```python
from build123d import *

# Parameters (mm, degrees)
SKETCH_1_R          = 23
SKETCH_1_R_2        = 20
EXTRUDE_1_DEPTH     = 20
SKETCH_2_W          = 10
SKETCH_2_H          = 19.630909826
CUT_EXTRUDE_1_DEPTH = 20
SKETCH_3_W          = 5
SKETCH_3_H          = 10
EXTRUDE_2_DEPTH     = 20
FILLET_1_R          = 2
SKETCH_4_R          = 2.15
CUT_EXTRUDE_2_DEPTH = 20
SKETCH_5_W          = 8
SKETCH_5_H          = 11
EXTRUDE_3_DEPTH     = 20
SKETCH_6_R          = 1.5
CUT_EXTRUDE_3_DEPTH = 23


with BuildPart() as part:
    # 草图1 → 凸台-拉伸1 (new body)
    with BuildSketch(Plane.XY):
        Circle(SKETCH_1_R)
        Circle(SKETCH_1_R_2, mode=Mode.SUBTRACT)
    extrude(amount=EXTRUDE_1_DEPTH)

    # 草图2 → 切除-拉伸1 (cut)
    with BuildSketch(Plane.XY.offset(20)):
        with Locations((0, -20)):
            Rectangle(SKETCH_2_W, SKETCH_2_H)
    extrude(amount=-CUT_EXTRUDE_1_DEPTH, mode=Mode.SUBTRACT)

    # 草图3 → 凸台-拉伸2 (add)
    with BuildSketch(Plane.XY.offset(20)):
        with Locations((-7.5, -24.364916731)):
            Rectangle(SKETCH_3_W, SKETCH_3_H)
        with Locations((7.5, -24.364916731)):
            Rectangle(SKETCH_3_W, SKETCH_3_H)
    extrude(amount=-EXTRUDE_2_DEPTH)

    # 圆角1
    fillet_1_edges = [part.edges().sort_by_distance(p)[0] for p in [
        (5, -19.364916731, 10),
        (-5, -19.364916731, 10),
    ]]
    fillet(fillet_1_edges, radius=FILLET_1_R)

    # 草图4 → 切除-拉伸2 (cut)
    with BuildSketch(Plane(origin=(10, 0, 0), x_dir=(0, 0, -1), z_dir=(1, 0, 0))):
        with Locations(Location((-15, -25.038615954, 0), (0, 0, 90))):
            Circle(SKETCH_4_R)
        with Locations(Location((-5, -25.038615954, 0), (0, 0, 90))):
            Circle(SKETCH_4_R)
    extrude(amount=-CUT_EXTRUDE_2_DEPTH, mode=Mode.SUBTRACT)

    # 草图5 → 凸台-拉伸3 (add)
    with BuildSketch(Plane(origin=(0, 0, 0), x_dir=(-1, 0, 0), z_dir=(0, 0, -1))):
        with Locations((0, 27.5)):
            Rectangle(SKETCH_5_W, SKETCH_5_H)
    extrude(amount=-EXTRUDE_3_DEPTH)

    # 草图6 → 切除-拉伸3 (cut)
    with BuildSketch(Plane(origin=(4, 0, 0), x_dir=(0, 0, -1), z_dir=(1, 0, 0))):
        with Locations(Location((-5, 28, 0), (0, 0, 90))):
            Circle(SKETCH_6_R)
        with Locations(Location((-15, 28, 0), (0, 0, 90))):
            Circle(SKETCH_6_R)
    extrude(amount=-CUT_EXTRUDE_3_DEPTH, mode=Mode.SUBTRACT)


solid = part.part
```
Source: CAD feature listing. Evaluate the final solid. Frame: model axes, mm. A direction names the side the tool comes from. Coordinates: 2 decimals unless noted, no trailing zeros. Order: outer loops, then holes, each group sorted by start corner. A loop starts at its lowest first (then second) coordinate and runs counter-clockwise, first axis right, second up. Notation, with made-up numbers: (78, -14) - (102, -14) arc R33 ccw to (102, 16) - close; hole circle Ø2 at (78, -28.75). An arc over 180 degrees is marked (long way). One line per item, written item: value.
1) Contact query for flat-ended pins moving along their axis: pin 1 (4.5 mm diameter, centred on y = -24, z = 6, fed in from +X); pin 2 (6 mm diameter, centred on x = 14, z = 3.5, fed in from -Y); pin 3 (2 mm diameter, centred on x = -7.5, y = -15.5, fed in from -Z); pin 4 (1 mm diameter, centred on y = -13, z = 10, fed in from -X). Output: stop coordinate, or through.
Computed values:
pin 1: stops at x = 10
pin 2: stops at y = -20.2
pin 3: passes through
pin 4: stops at x = -19.31
2) Cut plane B-B on y = 28. Output: boundary loops of the cut face in (x, z), plus the area to 3 significant figures.
Computed values:
outline: (-4, 0) - (4, 0) - (4, 3.5) - (-4, 3.5) - close; (-4, 6.5) - (4, 6.5) - (4, 13.5) - (-4, 13.5) - close; (-4, 16.5) - (4, 16.5) - (4, 20) - (-4, 20) - close
area: 112 mm^2
3) Reachability of faces 1 (the face through (10, -25, 10)), 2 (the face through (5, -25, 10)), 3 (the face through (-10, -25, 10)), 4 (the face through (4, 28, 10)) from +Z, -Z, +X, -X, +Y, -Y: full face, straight path, thin tool, end or side. Return the list, or none.
Computed values:
face 1: +Z, -Z, +X, -Y
face 2: +Z, -Z, -Y
face 3: +Z, -Z, -X, -Y
face 4: +Z, -Z, +X, +Y
4) Cut plane D-D on y = 0. Output: boundary loops of the cut face in (x, z), plus the area to 3 significant figures.
Computed values:
outline: (-23, 0) - (-20, 0) - (-20, 20) - (-23, 20) - close; (20, 0) - (23, 0) - (23, 20) - (20, 20) - close
area: 120 mm^2
5) Cut plane A-A on z = 5. Output: boundary loops of the cut face in (x, y).
Computed values:
outline: (-10, -29.36) - (-5, -29.36) - (-5, -27.19) - (-10, -27.19) - close; (-10, -22.89) - (-5, -22.89) - (-5, -20.86) arc R2 ccw to (-6.36, -18.96) arc R20 cw (long way) to (6.36, -18.96) arc R2 ccw to (5, -20.86) - (5, -22.89) - (10, -22.89) - (10, -20.71) arc R23 ccw to (4, 22.65) - (4, 26.5) - (-4, 26.5) - (-4, 22.65) arc R23 ccw to (-10, -20.71) - close; (-4, 29.5) - (4, 29.5) - (4, 33) - (-4, 33) - close; (5, -29.36) - (10, -29.36) - (10, -27.19) - (5, -27.19) - close
6) Ray query, line 1 (Z direction, x = 0, y = 28); line 2 (X direction, y = -21, z = 8.25); line 3 (Y direction, x = -15, z = 10.5). Return the intervals inside material, ascending. Write a range as [from, to].
Computed values:
line 1: z = [0, 3.5], [6.5, 13.5], [16.5, 20]
line 2: x = [-10, -5], [5, 10]
line 3: y = [-17.44, -13.23], [13.23, 17.44]
7) Cut plane C-C on x = 0. Output: boundary loops of the cut face in (y, z).
Computed values:
outline: (20, 0) - (33, 0) - (33, 20) - (20, 20) - close; hole circle Ø3 at (28, 5); hole circle Ø3 at (28, 15)
8) Mould query, pull axis Z, two halves, no side actions, for faces 5 (the face through (-0.1, 20.4, 20)), 6 (the face through (7, -29.365, 10)), 7 (the face through (7.535, -27.187, 5.095)). Classes: released by +Z, released by -Z, zero draft, split by the parting line, or undercut.
Computed values:
face 5: released by +Z
face 6: zero draft
face 7: undercut
